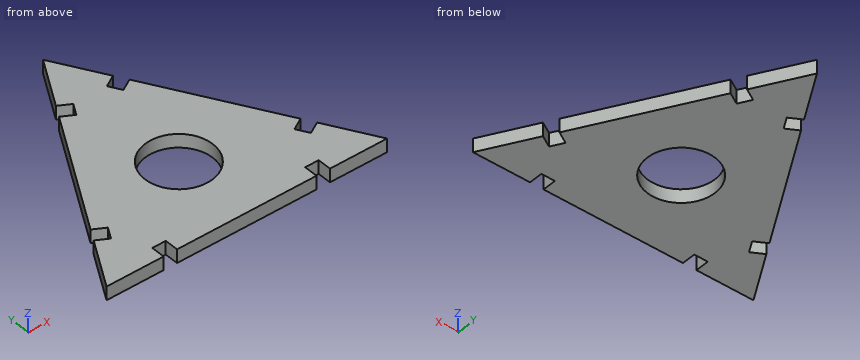
Autodesk Inventor part; units mm, degrees
ref_plane "YZ Plane" through (0, 0, 0) normal (1, 0, 0) x (0, 1, 0)
ref_plane "XZ Plane" through (0, 0, 0) normal (0, 1, 0) x (-1, 0, 0)
ref_plane "XY Plane" through (0, 0, 0) normal (0, 0, 1) x (1, 0, 0)
sketch "Sketch1" plane through (0, 0, 0) normal (0, 0, 1) x (1, 0, 0)
  circle A0 centre (0, 0) radius 7.5
  line L0 (31.1769, -18) -> (-31.1769, -18) construction
  line L1 (-31.1769, -18) -> (0, 36) construction
  line L2 (0, 36) -> (31.1769, -18) construction
  line L3 (15.5, -18) -> (15.5, -15)
  line L4 (15.5, -15) -> (18.5, -15)
  line L5 (18.5, -15) -> (18.5, -18)
  line L6 (-18.5, -18) -> (-18.5, -15)
  line L7 (-18.5, -15) -> (-15.5, -15)
  line L8 (-15.5, -15) -> (-15.5, -18)
  line L9 (-31.1769, -18) -> (15.5885, 9) construction
  line L10 (31.1769, -18) -> (-15.5885, 9) construction
  line L11 (0, 36) -> (0, -18) construction
  line L12 (6.3385, 25.0215) -> (3.7404, 23.5215)
  line L13 (3.7404, 23.5215) -> (5.2404, 20.9234)
  line L14 (5.2404, 20.9234) -> (7.8385, 22.4234)
  line L15 (23.3385, -4.4234) -> (20.7404, -5.9234)
  line L16 (20.7404, -5.9234) -> (22.2404, -8.5215)
  line L17 (22.2404, -8.5215) -> (24.8385, -7.0215)
  line L18 (-24.8385, -7.0215) -> (-22.2404, -8.5215)
  line L19 (-22.2404, -8.5215) -> (-20.7404, -5.9234)
  line L20 (-20.7404, -5.9234) -> (-23.3385, -4.4234)
  line L21 (-7.8385, 22.4234) -> (-5.2404, 20.9234)
  line L22 (-5.2404, 20.9234) -> (-3.7404, 23.5215)
  line L23 (-3.7404, 23.5215) -> (-6.3385, 25.0215)
  line L24 (-6.3385, 25.0215) -> (0, 36)
  line L25 (6.3385, 25.0215) -> (0, 36)
  line L26 (7.8385, 22.4234) -> (23.3385, -4.4234)
  line L27 (24.8385, -7.0215) -> (31.1769, -18)
  line L28 (31.1769, -18) -> (18.5, -18)
  line L29 (15.5, -18) -> (-15.5, -18)
  line L30 (-18.5, -18) -> (-31.1769, -18)
  line L31 (-31.1769, -18) -> (-24.8385, -7.0215)
  line L32 (-23.3385, -4.4234) -> (-7.8385, 22.4234)
  dimension "d3" = 15
  dimension "d4" = 18.5
  dimension "d5" = 18.5
  dimension "d8" = 3
  dimension "d9" = 18
  dimension "d10" = 3
  dimension "d11" = 3
  dimension "d12" = 18.5
  dimension "d13" = 3
  dimension "d14" = 3
  dimension "d15" = 18.5
  dimension "d16" = 3
  dimension "d17" = 3
  dimension "d18" = 18.5
  dimension "d19" = 3
  dimension "d20" = 3
  dimension "d21" = 3
  dimension "d22" = 18.5
  dimension "d23" = 3
extrude "Extrusion2" add sketch "Sketch1" along normal blind 3
equation "\"d11\" = d10"
equation "\"d12\" = d4"
equation "\"d13\" = d10"
equation "\"d14\" = d8"
equation "\"d15\" = d4"
equation "\"d16\" = d13"
equation "\"d17\" = d8"
equation "\"d18\" = d4"
equation "\"d19\" = d10"
equation "\"d20\" = d8"
equation "\"d21\" = d8"
equation "\"d22\" = d4"
equation "\"d23\" = d10"
properties part number "actuator"
Input: part model. Units: mm. Frame: model coordinates. Give positions to 0.01 mm unless a question says otherwise; leave off trailing zeros. Write each loop counter-clockwise with the first axis right and the second up, starting at its lowest first coordinate (ties: lowest second). Pieces come first, ordered by that corner, then holes. Notation, with made-up numbers: M 13,34 L 18,34 A19 ccw 18,67 Z; hole C 70,15 d1. An arc over 180 degrees is marked long. Write item = value, one per line. Start each with the question number.
1) Cut plane A-A on z = 1.25. Return the cut outline in (x, y), then the cut area to 3 significant figures.
2) Material intervals for line 1 along Y through (x, z) = (21, 1.55); line 2 along Y through (x, z) = (-22, 0.95); line 3 along Y through (x, z) = (-9, 2.55), sorted ascending. Write a range as [from, to].
3) Cut plane C-C on x = -11. Return the cut outline in (y, z).
4) Cut plane D-D on y = 11. Return the cut outline in (x, z).
5) Cut plane B-B on y = 0. Return the cut outline in (x, z).
6) First-contact query: pin 1 Ø1.5 at (y, z) = (-16.5, 1) entering from -X; pin 2 Ø1.5 at (y, z) = (10.5, 2.5) entering from -X; pin 3 Ø1.5 at (x, z) = (-17.5, 2) entering from -Y. Flat tips, straight axial feed; report the tip coordinate or a pass-through.
Solved:
q1.outline = M -31.18,-18 L -18.5,-18 L -18.5,-15 L -15.5,-15 L -15.5,-18 L 15.5,-18 L 15.5,-15 L 18.5,-15 L 18.5,-18 L 31.18,-18 L 24.84,-7.02 L 22.24,-8.52 L 20.74,-5.92 L 23.34,-4.42 L 7.84,22.42 L 5.24,20.92 L 3.74,23.52 L 6.34,25.02 L 0,36 L -6.34,25.02 L -3.74,23.52 L -5.24,20.92 L -7.84,22.42 L -23.34,-4.42 L -20.74,-5.92 L -22.24,-8.52 L -24.84,-7.02 Z; hole C 0,0 d15
q1.area = 1,450 mm2
q2.line_1 = [-18, -6.37], [-5.77, -0.37]
q2.line_2 = [-18, -8.11], [-5.2, -2.11]
q2.line_3 = [-18, 20.41]
q3.outline = M -18,0 L 16.95,0 L 16.95,3 L -18,3 Z
q4.outline = M -14.43,0 L 14.43,0 L 14.43,3 L -14.43,3 Z
q5.outline = M -20.78,0 L -7.5,0 L -7.5,3 L -20.78,3 Z; M 7.5,0 L 20.78,0 L 20.78,3 L 7.5,3 Z
q6.pin_1 = -30.74
q6.pin_2 = -15.16
q6.pin_3 = -15
